from build123d import *

# Parameters (mm, degrees)
BOSS_EXTRU_2_DEPTH      = 1
BOSS_EXTRU_2_DEPTH_BACK = 1
ESQUISSE3_R             = 0.625
ENL_V_MAT_EXTRU_1_DEPTH = 10


with BuildPart() as part:
    # Esquisse1 → Boss.-Extru.2 (new, two sides: drawn at the far end of the back side and taken through both)
    with BuildSketch(Plane.XY.offset(-BOSS_EXTRU_2_DEPTH_BACK)):
        with BuildLine():
            Line((0, 0), (9, 0))
            Line((9, 0), (9, 12))
            Line((9, 12), (5.5, 12))
            Line((5.5, 12), (5.5, 9))
            Line((5.5, 9), (2.5, 9))
            Line((2.5, 9), (2.5, 12))
            Line((2.5, 12), (-1, 12))
            Line((-1, 12), (-1, 4.358898944))
            ThreePointArc((-1, 4.358898944), (-0.253205655, 2.236067977), (0, 0))
        make_face()
    extrude(amount=BOSS_EXTRU_2_DEPTH + BOSS_EXTRU_2_DEPTH_BACK)

    # Esquisse3 → Enlèv. mat.-Extru.1 (cut)
    with BuildSketch(Plane.XY.offset(1)):
        with Locations((2, 3)):
            Circle(ESQUISSE3_R)
        with Locations((6, 3)):
            Circle(ESQUISSE3_R)
    extrude(amount=-ENL_V_MAT_EXTRU_1_DEPTH, mode=Mode.SUBTRACT)


solid = part.part
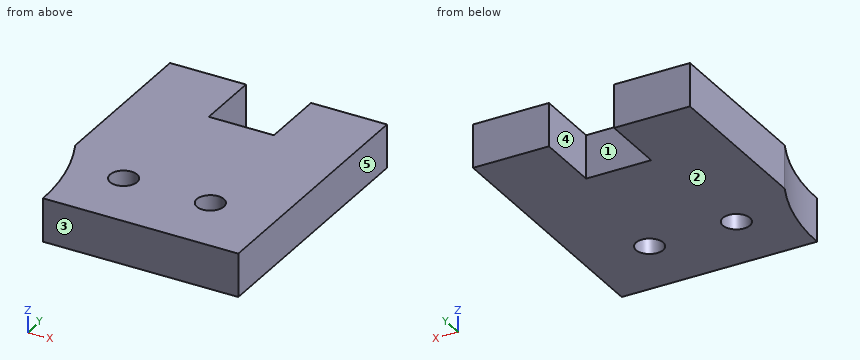
Design review of the part built by this model. Coordinates are the model's own, in mm. Face numbers are marked on the shaded views. A direction names the side the tool comes from. Round coordinates to 2 decimals unless told otherwise and drop trailing zeros. Loops run counter-clockwise (first coordinate to the right, second up) from the corner with the lowest first, then second, coordinate; pieces in that order, holes last. Notation, with made-up numbers: (82.5, 20.5) - (112.5, 20.5) arc R6 ccw to (112.5, 31.5) - close; hole circle Ø4 at (-27, 76.5). An arc over 180 degrees is marked (long way). One line per item, written item: value. Start each with the question number.
1) Consider section D-D on y = 3. Give the boundary of the cut face in (x, z) (3 decimals).
2) Draft analysis for pull direction X (two halves, no side actions). For the marked faces 3, 4 and 5, state which applies: +X half, -X half, draft (parallel to the pull), parting line (faces both ways), or undercut.
3) For the marked faces 1 and 2, list the 3-axis set-ups (+Z, -Z, +X, -X, +Y, -Y) from which the entire face can be reached by the end or side of a thin tool; tool diameter is ignored.
4) To check wall thickness, follow L1, parallel to Y at x = 2, z = -0.2 (3 decimals); L2, parallel to X at y = 10.25, z = 0.6; L3, parallel to Y at x = 4, z = 0.1. State the ranges of each line that lie inside material, in increasing order. Write a range as from..to.
5) Consider section A-A on y = 9.75. Give the boundary of the cut face in (x, z).
6) Consider section B-B on z = -0.3. Give the boundary of the cut face in (x, y) (3 decimals).
7) Consider section C-C on x = 2. Give the boundary of the cut face in (y, z) (3 decimals).
Reported:
1. outline: (-0.461, -1) - (1.375, -1) - (1.375, 1) - (-0.461, 1) - close; (2.625, -1) - (5.375, -1) - (5.375, 1) - (2.625, 1) - close; (6.625, -1) - (9, -1) - (9, 1) - (6.625, 1) - close
2. face 3: draft
2. face 4: undercut
2. face 5: +X half
3. face 1: +Z, -Z, +Y
3. face 2: -Z, +X, -X, +Y, -Y
4. L1: y = 0..2.375, 3.625..12
4. L2: x = -1..2.5, 5.5..9
4. L3: y = 0..9
5. outline: (-1, -1) - (2.5, -1) - (2.5, 1) - (-1, 1) - close; (5.5, -1) - (9, -1) - (9, 1) - (5.5, 1) - close
6. outline: (-1, 4.359) arc R10 cw to (0, 0) - (9, 0) - (9, 12) - (5.5, 12) - (5.5, 9) - (2.5, 9) - (2.5, 12) - (-1, 12) - close; hole circle Ø1.25 at (2, 3); hole circle Ø1.25 at (6, 3)
7. outline: (0, -1) - (2.375, -1) - (2.375, 1) - (0, 1) - close; (3.625, -1) - (12, -1) - (12, 1) - (3.625, 1) - close
